Autodesk Inventor part; units mm, degrees
ref_plane "YZ Plane" through (0, 0, 0) normal (1, 0, 0) x (0, 1, 0)
ref_plane "XZ Plane" through (0, 0, 0) normal (0, 1, 0) x (-1, 0, 0)
ref_plane "XY Plane" through (0, 0, 0) normal (0, 0, 1) x (1, 0, 0)
sketch "Sketch1" plane through (0, 0, 0) normal (0, 0, 1) x (1, 0, 0)
  line L0 (-60.325, -53.975) -> (60.325, -53.975)
  line L1 (60.325, -53.975) -> (60.325, 53.975)
  line L2 (60.325, 53.975) -> (-60.325, 53.975)
  line L3 (-60.325, 53.975) -> (-60.325, -53.975)
  line L4 (-60.325, -53.975) -> (60.325, 53.975) construction
  line L5 (60.325, -53.975) -> (-60.325, 53.975) construction
  point P0 (0, 0)
  dimension "d0" = 120.65
  dimension "d1" = 107.95
extrude "Polycarbonate Plate" add sketch "Sketch1" along normal blind 12.7
sketch "Sketch2" plane through (0, 0, 12.7) normal (0, 0, 1) x (1, 0, 0)
  line L0 (-42.0687, -50.8) -> (44.2913, -50.8)
  line L1 (55.7212, -39.37) -> (55.7212, 39.37)
  line L2 (44.2912, 50.8) -> (-42.0687, 50.8)
  line L3 (-53.4987, 39.37) -> (-53.4987, -39.37)
  line L4 (-53.4987, -50.8) -> (55.7212, 50.8) construction
  line L5 (55.7212, -50.8) -> (-53.4987, 50.8) construction
  line L6 (-35.4647, 46.101) -> (37.6872, 46.101)
  line L7 (51.6573, 32.131) -> (51.6573, -32.131)
  line L8 (37.6874, -46.157) -> (-35.4649, -46.157)
  line L9 (-49.4347, -32.131) -> (-49.4347, 32.131)
  arc A0 (-51.9112, 50.8) -> (-53.4987, 49.2125) centre (-51.9112, 49.2125) ccw
  arc A1 (-35.4647, 46.101) -> (-49.4347, 32.131) centre (-35.4647, 32.131) ccw
  arc A2 (51.6573, 32.131) -> (37.6872, 46.101) centre (37.6872, 32.131) ccw
  arc A3 (37.6874, -46.157) -> (51.6573, -32.131) centre (37.6874, -32.187) ccw
  arc A4 (-49.4347, -32.131) -> (-35.4649, -46.157) centre (-35.4649, -32.187) ccw
  arc A5 (-42.0687, 50.8) -> (-53.4987, 39.37) centre (-42.0687, 39.37) ccw
  arc A6 (55.7212, 39.37) -> (44.2912, 50.8) centre (44.2912, 39.37) ccw
  arc A7 (44.2913, -50.8) -> (55.7212, -39.37) centre (44.2913, -39.37) ccw
  arc A8 (-53.4987, -39.37) -> (-42.0687, -50.8) centre (-42.0687, -39.37) ccw
  point P0 (1.1113, 0)
  dimension "d4" = 109.22
  dimension "d5" = 101.6
  dimension "d6" = 4.699
  dimension "d10" = 13.97
  dimension "d11" = 11.43
  dimension "d26" = 4.064
  dimension "d28" = 4.064
extrude "Lid Recess" cut sketch "Sketch2" against normal blind 6.35
sketch "Sketch3" plane through (0, 0, 0) normal (0, 0, -1) x (-1, 0, 0)
  line L0 (35.7188, -40.4812) -> (-35.7188, -40.4813)
  line L1 (-48.4187, -27.7813) -> (-48.4188, 27.7812)
  line L2 (-35.7188, 40.4812) -> (35.7187, 40.4812)
  line L3 (48.4188, 27.7812) -> (48.4188, -27.7812)
  line L4 (48.4188, -40.4812) -> (-48.4188, 40.4812) construction
  line L5 (-48.4188, -40.4813) -> (48.4188, 40.4813) construction
  line L6 (-43.3388, 23.9713) -> (-43.3388, -23.9713)
  line L7 (-31.9088, -35.4013) -> (31.9088, -35.4013)
  line L8 (43.3388, -23.9713) -> (43.3388, 23.9713)
  line L9 (31.9088, 35.4013) -> (-31.9088, 35.4013)
  arc A0 (-43.3388, -23.9713) -> (-31.9088, -35.4013) centre (-31.9088, -23.9713) ccw
  arc A1 (31.9088, -35.4013) -> (43.3388, -23.9713) centre (31.9088, -23.9713) ccw
  arc A2 (43.3388, 23.9713) -> (31.9088, 35.4013) centre (31.9088, 23.9713) ccw
  arc A3 (-31.9088, 35.4013) -> (-43.3388, 23.9713) centre (-31.9088, 23.9713) ccw
  arc A4 (-35.7188, 40.4812) -> (-48.4188, 27.7812) centre (-35.7188, 27.7812) ccw
  arc A5 (-48.4187, -27.7813) -> (-35.7188, -40.4813) centre (-35.7188, -27.7813) ccw
  arc A6 (35.7188, -40.4812) -> (48.4188, -27.7812) centre (35.7188, -27.7812) ccw
  arc A7 (48.4188, 27.7812) -> (35.7187, 40.4812) centre (35.7188, 27.7812) ccw
  point P0 (0, 0)
  dimension "d14" = 96.8375
  dimension "d15" = 80.9625
  dimension "d16" = 5.08
  dimension "d17" = 11.43
  dimension "d18" = 12.7
fillet "Fillet1" radius 3.175 4 edges at (-60.325, 53.975, 6.35) (-60.325, -53.975, 6.35) (60.325, 53.975, 6.35) (60.325, -53.975, 6.35)
extrude "Small Recess" cut sketch "Sketch3" against normal blind 6.35
sketch "Sketch4" plane through (0, 0, 0) normal (0, 0, -1) x (-1, 0, 0)
  line L0 (-31.6778, 32.3024) -> (31.6778, 32.3024)
  line L1 (31.6778, 32.3024) -> (31.6778, -32.3024)
  line L2 (31.6778, -32.3024) -> (-31.6778, -32.3024)
  line L3 (-31.6778, -32.3024) -> (-31.6778, 32.3024)
  line L4 (-31.6778, 32.3024) -> (31.6778, -32.3024) construction
  line L5 (31.6778, 32.3024) -> (-31.6778, -32.3024) construction
  point P0 (0, 0)
extrude "Inside Dimension" cut sketch "Sketch4" against normal through all
fillet "Fillet2" radius 6.35 4 edges at (-31.6778, 32.3024, 6.35) (31.6778, -32.3024, 6.35) (31.6778, 32.3024, 6.35) (-31.6778, -32.3024, 6.35)
fillet "Fillet3" radius 3.175 8 edges at (-29.8179, -30.4425, 0) (0, -32.3024, 0) (29.8179, -30.4425, 0) (31.6778, 0, 0) (29.8179, 30.4425, 0) (0, 32.3024, 0) (-29.8179, 30.4425, 0) (-31.6778, 0, 0)
sketch "Sketch5" plane through (0, 0, 12.7) normal (0, 0, 1) x (1, 0, 0)
  arc A0 (57.15, -53.975) -> (60.325, -50.8) centre (57.15, -50.8) ccw
  line L0 (60.325, -50.8) -> (60.325, 50.8)
  arc A1 (60.325, 50.8) -> (57.15, 53.975) centre (57.15, 50.8) ccw
  arc A2 (-57.15, 53.975) -> (-60.325, 50.8) centre (-57.15, 50.8) ccw
  line L1 (-60.325, 50.8) -> (-60.325, -50.8)
  arc A3 (-60.325, -50.8) -> (-57.15, -53.975) centre (-57.15, -50.8) ccw
  line L2 (57.15, 53.975) -> (57.15, -53.975)
  line L3 (-57.15, -53.975) -> (-57.15, 53.975)
extrude "Extrusion5" cut sketch "Sketch5" against normal through all
fillet "Fillet4" radius 9.525 4 edges at (-57.15, 53.975, 6.35) (57.15, 53.975, 6.35) (57.15, -53.975, 6.35) (-57.15, -53.975, 6.35)
sketch "Sketch6" plane through (0, 0, 12.7) normal (0, 0, 1) x (1, 0, 0)
  arc A0 (-49.4347, -32.131) -> (-35.4649, -46.157) centre (-35.4649, -32.187) ccw
  line L0 (-35.4649, -46.157) -> (37.6874, -46.157)
  arc A1 (37.6874, -46.157) -> (51.6573, -32.131) centre (37.6874, -32.187) ccw
  line L1 (51.6573, -32.131) -> (51.6573, 32.131)
  arc A2 (51.6573, 32.131) -> (37.6872, 46.101) centre (37.6872, 32.131) ccw
  line L2 (37.6872, 46.101) -> (-35.4647, 46.101)
  arc A3 (-35.4647, 46.101) -> (-49.4347, 32.131) centre (-35.4647, 32.131) ccw
  line L3 (-49.4347, 32.131) -> (-49.4347, -32.131)
  arc A4 (-35.4647, 44.1873) -> (-47.521, 32.131) centre (-35.4647, 32.131) ccw
  line L4 (-35.4647, 44.1873) -> (37.6873, 44.1873)
  arc A5 (49.7435, 32.131) -> (37.6873, 44.1873) centre (37.6872, 32.131) ccw
  line L5 (49.7435, 32.131) -> (49.7435, -32.135)
  arc A6 (37.6874, -44.2432) -> (49.7435, -32.135) centre (37.6874, -32.187) ccw
  line L6 (37.6874, -44.2432) -> (-35.4649, -44.2432)
  arc A7 (-47.521, -32.135) -> (-35.4649, -44.2432) centre (-35.4649, -32.187) ccw
  line L7 (-47.521, -32.135) -> (-47.521, 32.131)
extrude "Extrusion6" cut sketch "Sketch6" against normal blind 3.175
equation "\"d28\" = d26"
properties material "POLYCARBONATE, CLEAR"
The model under review builds one solid part; all positions refer to its coordinate system, in mm. A direction names the side the tool comes from. Coordinates: 2 decimals unless noted, no trailing zeros. Write each loop counter-clockwise with the first axis right and the second up, starting at its lowest first coordinate (ties: lowest second). Pieces come first, ordered by that corner, then holes.
1) To check wall thickness, follow probe 1 along Y at (x, z) = (12, 11.5) (3 decimals); probe 2 along Y at (x, z) = (18.5, 7.75) (3 decimals); probe 3 along Y at (x, z) = (-32, 12) (3 decimals). State the ranges of each line that lie inside material, in increasing order.
2) Clearance check with a flat-ended pin moving along its axis: pin 1 Ø1 at (x, y) = (6, 36.5) entering from -Z. State where the tip first meets the part, or that it passes through.
3) We need section B-B on y = 38. State the section outline as (x, z) points (3 decimals).
4) The part is to be moulded in two halves that separate along X. For faces 4 (the face through (44.6, 36.86, 3.13)), 5 (the face through (39, 0, 0)), 6 (the face through (-54.434, -51.111, 6.439)), say which applies: pulls with the +X half, pulls with the -X half, needs draft (parallel to the pull), parting line crosses it, or undercut.
5) We need section C-C on x = -45. State the section outline as (y, z) points (3 decimals), then the cut area to 3 significant figures.
6) Machinability: for faces 1 (the face through (-29.87, -30.39, 8)), 2 (the face through (-32.63, -0.36, 0.91)), 3 (the face through (-43.896, 40.749, 11.135)), which of the approach directions +Z, -Z, +X, -X, +Y, -Y give a long, thin tool a straight path to every point of the face, cutting with its end or side? Answer none if there is none.
Answer list:
1. probe 1: y = -53.975 to -50.8, -44.243 to -32.302, 32.302 to 44.187, 50.8 to 53.975
1. probe 2: y = -53.975 to -50.8, -46.157 to -32.302, 32.302 to 46.101, 50.8 to 53.975
1. probe 3: y = -53.975 to -50.8, -44.243 to 44.187, 50.8 to 53.975
2. pin 1: stops at z = 6.35
3. outline: (-57.15, 0) - (-43.26, 0) - (-43.26, 6.35) - (43.26, 6.35) - (43.26, 0) - (57.15, 0) - (57.15, 12.7) - (55.721, 12.7) - (55.721, 6.35) - (50.365, 6.35) - (50.365, 9.525) - (48.219, 9.525) - (48.219, 12.7) - (-45.996, 12.7) - (-45.996, 9.525) - (-48.142, 9.525) - (-48.142, 6.35) - (-53.499, 6.35) - (-53.499, 12.7) - (-57.15, 12.7) - close
4. face 4: undercut
4. face 5: needs draft
4. face 6: pulls with the -X half
5. outline: (-53.975, 0) - (-36.45, 0) - (-36.45, 6.35) - (36.45, 6.35) - (36.45, 0) - (53.975, 0) - (53.975, 12.7) - (50.418, 12.7) - (50.418, 6.35) - (42.341, 6.35) - (42.341, 9.525) - (39.509, 9.525) - (39.509, 12.7) - (-39.565, 12.7) - (-39.565, 9.525) - (-42.397, 9.525) - (-42.397, 6.35) - (-50.418, 6.35) - (-50.418, 12.7) - (-53.975, 12.7) - close
5. area: 788 mm2
6. face 1: +Z, -Z
6. face 2: -Z
6. face 3: +Z
